```python
from build123d import *

# Parameters (mm, degrees)
SKETCH_1_W               = 70
SKETCH_1_H               = 20
EXTRUDE_1_DEPTH          = 11
SKETCH_3_W               = 70
SKETCH_3_H               = 15
EXTRUDE_2_DEPTH          = 25
CUT_EXTRUDE_1_DEPTH      = 15
SKETCH_5_R               = 4.5
CUT_EXTRUDE_2_DEPTH      = 30
SKETCH_11_R              = 2.6
CUT_EXTRUDE_7_DEPTH      = 6
SKETCH_12_W              = 12
SKETCH_12_H              = 5
CUT_EXTRUDE_8_DEPTH      = 25
SKETCH_8_R               = 2.4
CUT_EXTRUDE_5_DEPTH      = 31.5
CUT_EXTRUDE_5_DEPTH_BACK = 6.5
SKETCH_10_R              = 2.4
CUT_EXTRUDE_6_DEPTH      = 26
CUT_EXTRUDE_6_DEPTH_BACK = 12
FILLET_1_R               = 5
CHAMFER_1_SIZE           = 0.6
FILLET_2_R               = 2


with BuildPart() as part:
    # 草图1 → 凸台-拉伸1 (new body)
    with BuildSketch(Plane.XY):
        with Locations((21.875, 8.541666667)):
            Rectangle(SKETCH_1_W, SKETCH_1_H)
    extrude(amount=EXTRUDE_1_DEPTH)

    # 草图3 → 凸台-拉伸2 (add)
    with BuildSketch(Plane.XY.offset(11)):
        with Locations((21.875, 11.041666667)):
            Rectangle(SKETCH_3_W, SKETCH_3_H)
    extrude(amount=EXTRUDE_2_DEPTH)

    # 草图4 → 切除-拉伸1 (cut)
    with BuildSketch(Plane.XZ.offset(-3.541666667)):
        Polygon((-13.125, 36), (-13.125, 11), (-1.125, 36), align=None)
        Polygon((56.875, 11), (44.875, 36), (56.875, 36), align=None)
        Polygon((5.125, 11), (25.125, 11), (25.125, 21), (38.625, 21), (38.625, 30.5), (18.625, 30.5), (18.625, 21), (18.625, 20.5), (5.125, 20.5), align=None)
    extrude(amount=-CUT_EXTRUDE_1_DEPTH, mode=Mode.SUBTRACT)

    # 草图5 → 切除-拉伸2 (cut)
    with BuildSketch(Plane.XY.offset(36)):
        with Locations((-5.625, 8.541666667)):
            Circle(SKETCH_5_R)
        with Locations((49.375, 8.541666667)):
            Circle(SKETCH_5_R)
    extrude(amount=-CUT_EXTRUDE_2_DEPTH, mode=Mode.SUBTRACT)

    # 草图11 → 切除-拉伸7 (cut)
    with BuildSketch(Plane.XY.offset(6)):
        with Locations((-5.625, 8.541666667)):
            Circle(SKETCH_11_R)
        with Locations((49.375, 8.541666667)):
            Circle(SKETCH_11_R)
    extrude(amount=-CUT_EXTRUDE_7_DEPTH, mode=Mode.SUBTRACT)

    # 草图12 → 切除-拉伸8 (cut)
    with BuildSketch(Plane.XY.offset(36)):
        with Locations((-7.125, 6.041666667)):
            Rectangle(SKETCH_12_W, SKETCH_12_H)
        with Locations((50.875, 6.041666667)):
            Rectangle(SKETCH_12_W, SKETCH_12_H)
    extrude(amount=-CUT_EXTRUDE_8_DEPTH, mode=Mode.SUBTRACT)

    # 草图8 → 切除-拉伸5 (cut, two sides)
    with BuildSketch(Plane(origin=(0, 0, 30.5), x_dir=(-1, 0, 0), z_dir=(0, 0, -1))) as cut_extrude_5_sk:
        with Locations((-28.625, 8.541666667)):
            Circle(SKETCH_8_R)
    extrude(amount=CUT_EXTRUDE_5_DEPTH, mode=Mode.SUBTRACT)
    extrude(cut_extrude_5_sk.sketch, amount=-CUT_EXTRUDE_5_DEPTH_BACK, mode=Mode.SUBTRACT)

    # 草图10 → 切除-拉伸6 (cut, two sides)
    with BuildSketch(Plane.XY.offset(11)) as cut_extrude_6_sk:
        with Locations((15.125, 8.541666667)):
            Circle(SKETCH_10_R)
    extrude(amount=CUT_EXTRUDE_6_DEPTH, mode=Mode.SUBTRACT)
    extrude(cut_extrude_6_sk.sketch, amount=-CUT_EXTRUDE_6_DEPTH_BACK, mode=Mode.SUBTRACT)

    # 圆角1
    fillet_1_edges = [part.edges().sort_by_distance(p)[0] for p in [
        (56.875, -1.458333333, 5.5),
        (-13.125, -1.458333333, 5.5),
    ]]
    fillet(fillet_1_edges, radius=FILLET_1_R)

    # 倒角1
    chamfer_1_edges = [part.edges().sort_by_distance(p)[0] for p in [
        (21.875, 18.541666667, 36),
        (-13.125, 18.541666667, 5.5),
        (56.875, 18.541666667, 5.5),
        (-7.125, 18.541666667, 23.5),
        (50.875, 18.541666667, 23.5),
        (5.125, 18.541666667, 15.75),
        (11.875, 18.541666667, 20.5),
        (18.625, 18.541666667, 25.5),
        (21.875, 18.541666667, 0),
        (28.625, 18.541666667, 30.5),
        (38.625, 18.541666667, 25.75),
        (31.875, 18.541666667, 21),
        (25.125, 18.541666667, 16),
        (15.125, 18.541666667, 11),
    ]]
    chamfer(chamfer_1_edges, length=CHAMFER_1_SIZE)

    # 圆角2
    fillet_2_edges = [part.edges().sort_by_distance(p)[0] for p in [
        (-1.125, 3.541666667, 23.5),
        (44.875, 3.541666667, 23.5),
        (25.125, 3.541666667, 16),
        (18.625, 3.541666667, 25.5),
    ]]
    fillet(fillet_2_edges, radius=FILLET_2_R)


solid = part.part
```
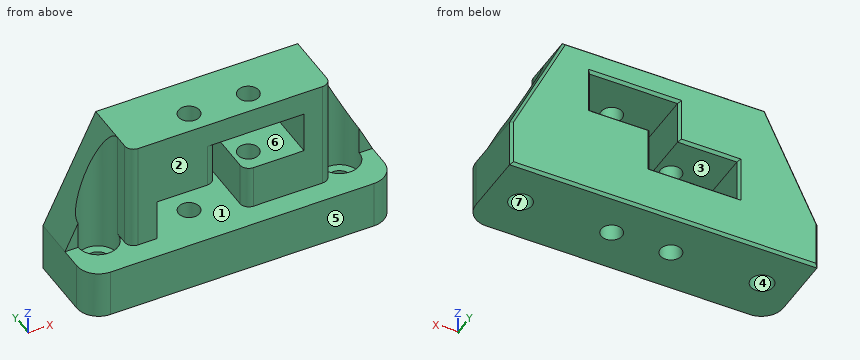
Build history of the part. All positions in model axes, mm. Face numbers are marked on the shaded views. A direction names the side the tool comes from. Round coordinates to 2 decimals unless told otherwise and drop trailing zeros. Write each loop counter-clockwise with the first axis right and the second up, starting at its lowest first coordinate (ties: lowest second). Pieces come first, ordered by that corner, then holes. Notation, with made-up numbers: (-26.75, 62) -> (11.25, 62) arc R28 ccw to (11.25, 82) -> close; hole circle Ø8 at (78.5, 77). An arc over 180 degrees is marked (long way). Put each result on its own line as item: value.
Item 1: Slice it at A-A, the plane y = 16.25. Give the cut face in (x, z) (3 decimals), plus the area to 3 significant figures.
Here are the results:
outline: (-13.125, 0) -> (56.875, 0) -> (56.875, 11) -> (44.875, 36) -> (-1.125, 36) -> (-13.125, 11) -> close; hole (5.125, 11) -> (25.125, 11) -> (25.125, 21) -> (38.625, 21) -> (38.625, 30.5) -> (18.625, 30.5) -> (18.625, 20.5) -> (5.125, 20.5) -> close
area: 1,840 mm^2
Item 2: Slice it at C-C, the plane x = 40.5. Give the cut face in (y, z), plus the area to 3 significant figures.
Here are the results:
outline: (-1.46, 0) -> (17.94, 0) -> (18.54, 0.6) -> (18.54, 35.4) -> (17.94, 36) -> (3.54, 36) -> (3.54, 11) -> (-1.46, 11) -> close
area: 595 mm^2
Item 3: Slice it at B-B, the plane z = 27. Give the cut face in (x, y) (3 decimals).
Here are the results:
outline: (-5.445, 13.038) arc R4.5 cw to (-1.125, 8.542) -> (-1.125, 5.542) arc R2 ccw to (0.875, 3.542) -> (16.625, 3.542) arc R2 ccw to (18.625, 5.542) -> (18.625, 17.942) -> (18.025, 18.542) -> (-4.779, 18.542) -> (-5.445, 17.942) -> close; (38.625, 3.542) -> (42.875, 3.542) arc R2 ccw to (44.875, 5.542) -> (44.875, 8.542) arc R4.5 cw to (49.195, 13.038) -> (49.195, 17.942) -> (48.529, 18.542) -> (39.225, 18.542) -> (38.625, 17.942) -> close; hole circle Ø4.8 at (15.125, 8.542)
Item 4: Flat gauge pins, fed straight in: P1, Ø5, axis at y = 9.5, z = 14, coming from the -X side (3 decimals); P2, Ø3, axis at y = 11.5, z = 16, coming from the +X side (3 decimals); P3, Ø3.5, axis at y = 7.5, z = 26.5, coming from the -X side. Where does each tip first touch, or does it go through?
Here are the results:
P1: stops at x = -12.885
P2: stops at x = 55.195
P3: stops at x = -1.18
Item 5: Wall check: probe 1 along Z at (x, y) = (9, 6); probe 2 along Z at (x, y) = (36.5, 11.75); probe 3 along X at (y, z) = (9, 34.5). Give the ranges that are in metal, low to high. Write a range as from..to.
Here are the results:
probe 1: z = 0..11, 20.5..36
probe 2: z = 0..21, 30.5..36
probe 3: x = -1.15..12.77, 17.48..26.27, 30.98..44.9
Item 6: Tool access for the marked faces 1, 2 and 3: list every direction of +Z, -Z, +X, -X, +Y, -Y with a clear straight run to the whole face (end or side of a thin tool).
Here are the results:
face 1: -Y
face 2: +Z, +X, -X, -Y
face 3: +Y, -Y
Item 7: Two-plate mould, pull along Y, no slides. Class the marked faces 4, 5, 6 and 7: pulls with the +Y half, pulls with the -Y half, needs draft (parallel to the pull), parting line crosses it, or undercut.
Here are the results:
face 4: undercut
face 5: pulls with the -Y half
face 6: needs draft
face 7: undercut
Item 8: Slice it at D-D, the plane z = 8. Give the cut face in (x, y) (3 decimals), plus the area to 3 significant figures.
Here are the results:
outline: (-13.125, 3.542) arc R5 ccw to (-8.125, -1.458) -> (51.875, -1.458) arc R5 ccw to (56.875, 3.542) -> (56.875, 17.942) -> (56.275, 18.542) -> (-12.525, 18.542) -> (-13.125, 17.942) -> close; hole circle Ø9 at (-5.625, 8.542); hole circle Ø4.8 at (15.125, 8.542); hole circle Ø4.8 at (28.625, 8.542); hole circle Ø9 at (49.375, 8.542)
area: 1,230 mm^2
